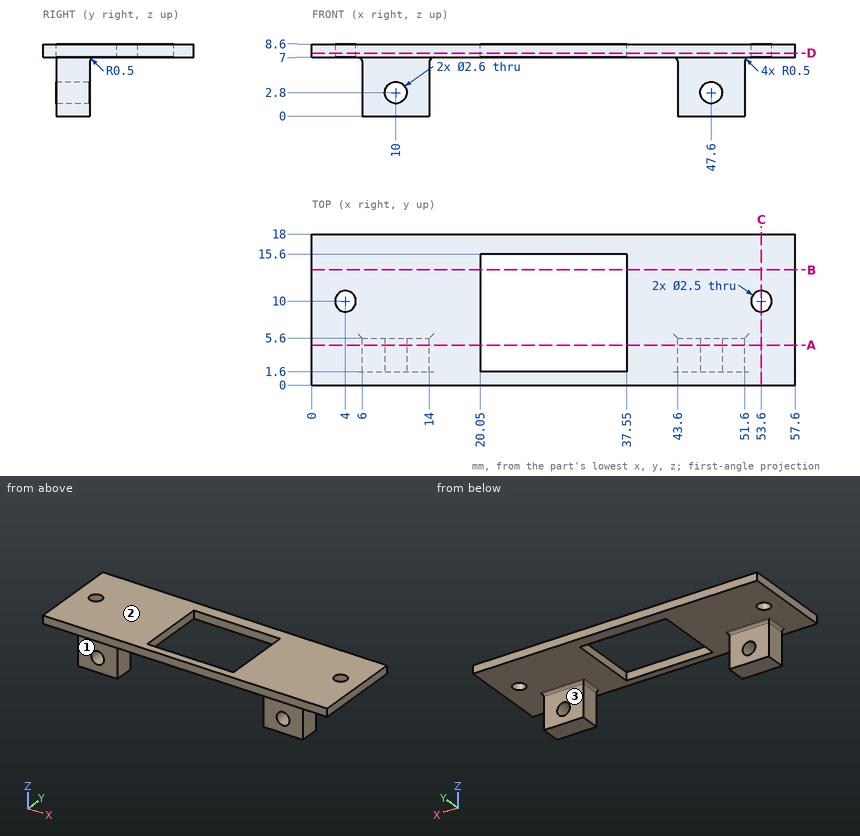
Print and shaded views of the part. All mm, measured from the part's lowest x, y and z. A direction names the side the tool comes from. Coordinates: 2 decimals unless noted, no trailing zeros. Loops run counter-clockwise (first coordinate to the right, second up) from the corner with the lowest first, then second, coordinate; pieces in that order, holes last. Notation, with made-up numbers: (-4.5, -8.75) -> (7.5, -8.75) arc R21 ccw to (7.5, 0.25) -> close; hole circle Ø2 at (42, -34). An arc over 180 degrees is marked (long way). Use a Markdown table: item, result. Add a question column.
Item 1: Band-saw the part on A-A on y = 4.75. Write the cut outline in (x, z).
Item 2: Probe probe 1 along X at (y, z) = (3.65, 2.8); probe 2 along X at (y, z) = (8.5, 8); probe 3 along Y at (x, z) = (53.6, 7.9). List the from-to ranges inside material, lowest first.
Item 3: Band-saw the part on B-B on y = 13.75. Write the cut outline in (x, z), plus the area to 3 significant figures.
Item 4: Which spindle directions (+Z, -Z, +X, -X, +Y, -Y) get a long thin tool onto all of the face, cutting with end or side? Do the marked faces 1, 2 and 3. Say none if no direction does.
Item 5: Band-saw the part on C-C on x = 53.6. Write the cut outline in (y, z).
Item 6: Flat gauge pins, fed straight in: P1, Ø1.2, axis at y = 3, z = 2.5, coming from the -X side; P2, Ø5.5, axis at x = 19.5, y = 9, coming from the -Z side; P3, Ø4, axis at x = 13.5, z = 3, coming from the +Y side. Where does each tip first touch, or does it go through?
Item 7: Band-saw the part on D-D on z = 7.5. Write the cut outline in (x, y), plus the area to 3 significant figures.
Geometry says:
| question | item | result |
|---|---|---|
| 1 | outline | (0, 7) -> (5.5, 7) arc R0.5 cw to (6, 6.5) -> (6, 0) -> (14, 0) -> (14, 6.5) arc R0.5 cw to (14.5, 7) -> (20.05, 7) -> (20.05, 8.6) -> (0, 8.6) -> close; (37.55, 7) -> (43.1, 7) arc R0.5 cw to (43.6, 6.5) -> (43.6, 0) -> (51.6, 0) -> (51.6, 6.5) arc R0.5 cw to (52.1, 7) -> (57.6, 7) -> (57.6, 8.6) -> (37.55, 8.6) -> close; hole circle Ø2.6 at (10, 2.8); hole circle Ø2.6 at (47.6, 2.8) |
| 2 | probe 1 | 6 to 8.7, 11.3 to 14, 43.6 to 46.3, 48.9 to 51.6 |
| 2 | probe 2 | 0 to 20.05, 37.55 to 57.6 |
| 2 | probe 3 | 0 to 8.75, 11.25 to 18 |
| 3 | outline | (0, 7) -> (20.05, 7) -> (20.05, 8.6) -> (0, 8.6) -> close; (37.55, 7) -> (57.6, 7) -> (57.6, 8.6) -> (37.55, 8.6) -> close |
| 3 | area | 64.2 mm² |
| 4 | face 1 | -Z, +X, -X, -Y |
| 4 | face 2 | +Z, +X, -X, +Y, -Y |
| 4 | face 3 | -Z, +X, -X, +Y |
| 5 | outline | (0, 7) -> (8.75, 7) -> (8.75, 8.6) -> (0, 8.6) -> close; (11.25, 7) -> (18, 7) -> (18, 8.6) -> (11.25, 8.6) -> close |
| 6 | P1 | x = 6 |
| 6 | P2 | z = 7 |
| 6 | P3 | y = 5.6 |
| 7 | outline | (0, 0) -> (57.6, 0) -> (57.6, 18) -> (0, 18) -> close; hole circle Ø2.5 at (4, 10); hole (20.05, 1.6) -> (37.55, 1.6) -> (37.55, 15.6) -> (20.05, 15.6) -> close; hole circle Ø2.5 at (53.6, 10) |
| 7 | area | 782 mm² |
